Design review of the part built by this model. Coordinates are the model's own, in mm. A direction names the side the tool comes from. Coordinates: 2 decimals unless noted, no trailing zeros. Write each loop counter-clockwise with the first axis right and the second up, starting at its lowest first coordinate (ties: lowest second). Pieces come first, ordered by that corner, then holes. Notation, with made-up numbers: (4.5, -11.5) - (62.5, -11.5) arc R21 cw to (62.5, 5.5) - close; hole circle Ø5 at (-17, -29). An arc over 180 degrees is marked (long way). Answer as CSV lines item,"result". Start each with the question number.
Q1. Machinability: for faces 1 (the face through (1940, 74.4, -33.2)), 2 (the face through (984, 76, -32.9)), which of the approach directions +Z, -Z, +X, -X, +Y, -Y give a long, thin tool a straight path to every point of the face, cutting with its end or side? Answer none if there is none.
Q2. We need section A-A (x = 227.5). Write out the cut boundary in (y, z).
Q3. We need section B-B (y = 78). Write out the cut boundary in (x, z), plus the area to 3 significant figures.
Q4. Clearance check with flat-ended pins moving along their axes: pin 1 (5 mm diameter, centred on x = 400, z = -16.95, fed in from -Y); pin 2 (1 mm diameter, centred on x = 1521.5, z = -9, fed in from +Y); pin 3 (5 mm diameter, centred on x = 679.5, y = 61.5, fed in from +Z). State where each tip first meets the part, or that it passes through.
Q5. For line 1 along X through (y, z) = (-0.4, -16.95); line 2 along Z through (x, y) = (1200, -0.6); line 3 along Z through (x, y) = (1792, 54), list the stretches that pass through material, from the lowest coordinate up. Write a range as [from, to].
from build123d import *

# Parameters (mm, degrees)
SKETCH2_W                    = 33.9
SKETCH2_H                    = 1
BASE_FLANGE1_DEPTH           = 1940
EDGE_FLANGE2_STRIP_W         = 5.4732
EDGE_FLANGE2_STRIP_H         = 1
EDGE_FLANGE2_STRIP_CUT_DEPTH = 1940
EDGE_FLANGE2_DEPTH           = 1940
SKETCH10_R                   = 3
CUT_EXTRUDE1_DEPTH           = 10
SKETCH10_3_R                 = 3
CUT_EXTRUDE2_DEPTH           = 10


# Sheet-metal steps are written as plain solids
with BuildPart() as part:
    # Sketch2 → Base-Flange1 (new body)
    with BuildSketch(Plane(origin=(0, 0, 0), x_dir=(0, 0, -1), z_dir=(1, 0, 0))):
        with Locations((16.95, -0.5)):
            Rectangle(SKETCH2_W, SKETCH2_H)
    extrude(amount=BASE_FLANGE1_DEPTH)

    # Edge-Flange2 strip (across the edge) → Edge-Flange2 strip cut (cut)
    with BuildSketch(Plane(origin=(1940, 0, -33.9), x_dir=(0, 0, 1), z_dir=(-1, 0, 0))):
        with Locations((-1, -0.5)):
            Rectangle(EDGE_FLANGE2_STRIP_W, EDGE_FLANGE2_STRIP_H)
    extrude(amount=EDGE_FLANGE2_STRIP_CUT_DEPTH, mode=Mode.SUBTRACT)

    # Edge-Flange2 section (across the edge) → Edge-Flange2 (add)
    with BuildSketch(Plane(origin=(1940, 0, -33.9), x_dir=(0, 0, 1), z_dir=(-1, 0, 0))):
        with BuildLine():
            Line((0, 0.7366), (0, 149))
            Line((0, 149), (1, 149))
            Line((1, 149), (1, 0.7366))
            ThreePointArc((1, 0.7366), (1.215745145, 0.215745145), (1.7366, 0))
            Line((1.7366, 0), (1.7366, -1))
            ThreePointArc((1.7366, -1), (0.508638364, -0.491361636), (0, 0.7366))
        make_face()
    extrude(amount=EDGE_FLANGE2_DEPTH)

    # Sketch10 → Cut-Extrude1 (cut)
    with BuildSketch(Plane(origin=(0, 0, 0), x_dir=(1, 0, 0), z_dir=(0, 1, 0))):
        with Locations(Location((800, 16.95, 0), (0, 0, 270))):
            Circle(SKETCH10_R)
    extrude(amount=-CUT_EXTRUDE1_DEPTH, mode=Mode.SUBTRACT)

    # Sketch10<3> → Cut-Extrude2 (cut)
    with BuildSketch(Plane(origin=(0, 0, 0), x_dir=(1, 0, 0), z_dir=(0, 1, 0))):
        with Locations(Location((400, 16.95, 0), (0, 0, 270))):
            Circle(SKETCH10_3_R)
        with Locations(Location((800, 16.95, 0), (0, 0, 270))):
            Circle(SKETCH10_3_R)
        with Locations(Location((1200, 16.95, 0), (0, 0, 270))):
            Circle(SKETCH10_3_R)
        with Locations(Location((1600, 16.95, 0), (0, 0, 270))):
            Circle(SKETCH10_3_R)
    extrude(amount=-CUT_EXTRUDE2_DEPTH, mode=Mode.SUBTRACT)


solid = part.part
Results list:
1,face 1,"+Z, -Z, +X, +Y, -Y"
1,face 2,"+Z, +X, -X, +Y"
2,outline,"(-1, -32.16) arc R1.74 ccw to (0.74, -33.9) - (149, -33.9) - (149, -32.9) - (0.74, -32.9) arc R0.74 cw to (0, -32.16) - (0, 0) - (-1, 0) - close"
3,outline,"(0, -33.9) - (1940, -33.9) - (1940, -32.9) - (0, -32.9) - close"
3,area,"1,940 mm2"
4,pin 1,"passes through"
4,pin 2,"stops at y = 0"
4,pin 3,"stops at z = -32.9"
5,line 1,"x = [0, 397], [403, 797], [803, 1197], [1203, 1597], [1603, 1940]"
5,line 2,"z = [-33.27, -19.95], [-13.95, 0]"
5,line 3,"z = [-33.9, -32.9]"
